from build123d import *

# Parameters (mm, degrees)
F1_DEPTH       = 15
F3_D           = 4
F3_CSINK_D     = 7
F3_CSINK_ANGLE = 90
F4_R           = 5


with BuildPart() as f1:
    # F0 (on Top) → F1 (new body)
    with BuildSketch(Plane.XY):
        with BuildLine():
            ThreePointArc((-10.0704716871, 5.3), (-9.3541459143, 6.4810766246), (-8.5, 7.5666637298))
            Line((-8.5, 7.5666637298), (-8.5, 8.5))
            Line((-8.5, 8.5), (-18.88, 8.5))
            Line((-18.88, 8.5), (-18.88, 5.3))
            Line((-18.88, 5.3), (-11.38, 5.3))
            Line((-11.38, 5.3), (-10.0704716871, 5.3))
        make_face()
        with BuildLine():
            ThreePointArc((-11.38, 0), (-11.0477682769, 2.7296915761), (-10.0704716871, 5.3))
            Line((-10.0704716871, 5.3), (-11.38, 5.3))
            Line((-11.38, 5.3), (-11.38, 0))
        make_face()
        with BuildLine():
            ThreePointArc((8.5, 0), (0, -8.5), (-8.5, 0))
            Line((-8.5, 0), (-8.5, 5.3))
            Line((-8.5, 5.3), (-10.0704716871, 5.3))
            ThreePointArc((-10.0704716871, 5.3), (-11.0477682769, 2.7296915761), (-11.38, 0))
            ThreePointArc((-11.38, 0), (0, -11.38), (11.38, 0))
            ThreePointArc((11.38, 0), (11.0477682769, 2.7296915761), (10.0704716871, 5.3))
            Line((10.0704716871, 5.3), (8.5, 5.3))
            Line((8.5, 5.3), (8.5, 0))
        make_face()
        with BuildLine():
            Line((11.38, 5.3), (10.0704716871, 5.3))
            ThreePointArc((10.0704716871, 5.3), (11.0477682769, 2.7296915761), (11.38, 0))
            Line((11.38, 0), (11.38, 5.3))
        make_face()
        with BuildLine():
            Line((8.5, 8.5), (8.5, 7.5666637298))
            ThreePointArc((8.5, 7.5666637298), (9.3541459143, 6.4810766246), (10.0704716871, 5.3))
            Line((10.0704716871, 5.3), (11.38, 5.3))
            Line((11.38, 5.3), (18.88, 5.3))
            Line((18.88, 5.3), (18.88, 8.5))
            Line((18.88, 8.5), (8.5, 8.5))
        make_face()
        with BuildLine():
            Line((-10.0704716871, 5.3), (-8.5, 5.3))
            Line((-8.5, 5.3), (-8.5, 7.5666637298))
            ThreePointArc((-8.5, 7.5666637298), (-9.3541459143, 6.4810766246), (-10.0704716871, 5.3))
        make_face()
        with BuildLine():
            Line((8.5, 7.5666637298), (8.5, 5.3))
            Line((8.5, 5.3), (10.0704716871, 5.3))
            ThreePointArc((10.0704716871, 5.3), (9.3541459143, 6.4810766246), (8.5, 7.5666637298))
        make_face()
    extrude(amount=F1_DEPTH)

    # F3 (through all)
    with Locations(Plane.XZ.offset(-5.3)):
        with Locations((-15.13, 7.5), (15.13, 7.5)):
            CounterSinkHole(F3_D / 2, F3_CSINK_D / 2, counter_sink_angle=F3_CSINK_ANGLE)

    # F4
    f4_edges = [f1.edges().sort_by_distance(p)[0] for p in [
        (-18.88, 6.9, 15),
        (-18.88, 6.9, 0),
        (18.88, 6.9, 15),
        (18.88, 6.9, 0),
    ]]
    fillet(f4_edges, radius=F4_R)


solid = f1.part
Here's how the part is built. I have some questions about the finished solid (model axes, mm). A direction names the side the tool comes from. Coordinates: 2 decimals unless noted, no trailing zeros. Write each loop counter-clockwise with the first axis right and the second up, starting at its lowest first coordinate (ties: lowest second). Pieces come first, ordered by that corner, then holes.
1) I'm going to push flat-ended pins straight in: pin 1 (4 mm diameter, centred on y = 2, z = 7, fed in from -X); pin 2 (6 mm diameter, centred on x = -8.5, z = 9, fed in from -Y); pin 3 (3.5 mm diameter, centred on x = -13.5, z = 10, fed in from -Y); pin 4 (5 mm diameter, centred on y = 4.5, z = 6, fed in from +X). Where does each tip first touch, or does it pass through?
Filled in:
pin 1: stops at x = -11.38
pin 2: stops at y = -9.96
pin 3: stops at y = 5.3
pin 4: stops at x = 18.88
2) If we section it at C-C (y = -0.5): List the corners of the cut face in (x, z) for me.
Filled in:
outline: (-11.37, 0) - (-8.49, 0) - (-8.49, 15) - (-11.37, 15) - close; (8.49, 0) - (11.37, 0) - (11.37, 15) - (8.49, 15) - close
3) Which directions (+Z, -Z, +X, -X, +Y, -Y) give clear straight access to the entire face, cutting with the end or side of a thin tool? Please do faces 4 (the face through (-14, 5.3, 4)), 5 (the face through (-17.45, 6.88, 1.5)), 6 (the face through (8.5, 4, 7)), 7 (the face through (11.38, 3, 7)).
Filled in:
face 4: +Z, -Z, -X, -Y
face 5: -Z, -X, +Y, -Y
face 6: +Z, -Z, +Y
face 7: +Z, -Z, +X, -Y
4) If we section it at D-D (y = -2.5): List the corners of the cut face in (x, z) for me, plus the area to 3 significant figures.
Filled in:
outline: (-11.1, 0) - (-8.12, 0) - (-8.12, 15) - (-11.1, 15) - close; (8.12, 0) - (11.1, 0) - (11.1, 15) - (8.12, 15) - close
area: 89.3 mm2
5) Thinking about a two-plate mould opening in Z: for faces 1 (the face through (-17.038, 7.662, 8.101)), 2 (the face through (17.45, 6.92, 1.5)), 3 (the face through (-8.5, 4, 7)), which applies, +Z half, -Z half, draft (parallel to the pull), parting line (faces both ways), or undercut?
Filled in:
face 1: undercut
face 2: -Z half
face 3: draft
6) If I drill on line 1 (X direction, y = 8, z = 7.5); line 2 (X direction, y = 0.5, z = 11.75); line 3 (Y direction, x = -14.5, z = 11.5), over which ranges is the centre line in solid material (lowest first)?
Filled in:
line 1: x = -18.88 to -17.13, -13.13 to -8.5, 8.5 to 13.13, 17.13 to 18.88
line 2: x = -11.38 to -8.5, 8.5 to 11.38
line 3: y = 5.3 to 8.5
7) If we section it at B-B (x = -15.13): List the corners of the cut face in (y, z) for me.
Filled in:
outline: (5.3, 0.16) - (8.5, 0.16) - (8.5, 5.5) - (6.8, 5.5) - (5.3, 4) - close; (5.3, 11) - (6.8, 9.5) - (8.5, 9.5) - (8.5, 14.84) - (5.3, 14.84) - close
8) If we section it at A-A (z = 7.5): List the corners of the cut face in (x, y) for me.
Filled in:
outline: (-18.88, 5.3) - (-18.63, 5.3) - (-17.13, 6.8) - (-17.13, 8.5) - (-18.88, 8.5) - close; (-13.13, 6.8) - (-11.63, 5.3) - (-11.38, 5.3) - (-11.38, 0) arc R11.38 ccw to (11.38, 0) - (11.38, 5.3) - (11.63, 5.3) - (13.13, 6.8) - (13.13, 8.5) - (8.5, 8.5) - (8.5, 0) arc R8.5 cw to (-8.5, 0) - (-8.5, 8.5) - (-13.13, 8.5) - close; (17.13, 6.8) - (18.63, 5.3) - (18.88, 5.3) - (18.88, 8.5) - (17.13, 8.5) - close
